Geometry check sheet. Reference: the model listing, model coordinates, mm. Round coordinates to 2 decimals unless told otherwise and drop trailing zeros. Order: outer loops, then holes, each group sorted by start corner. A loop starts at its lowest first (then second) coordinate and runs counter-clockwise, first axis right, second up.
(1) Sectioned sample at A-A (y = 0). Record the boundary of the cut face in (x, z).
(2) Sectioned sample at C-C (z = 2.05). Record the boundary of the cut face in (x, y), plus the area to 3 significant figures.
(3) Release check for a two-part mould opening along Y. For faces 1 (the face through (88.8, 3.4, 4)), 2 (the face through (86, 0, 3)), 3 (the face through (89, 0, 1)), 4 (the face through (180, 0, 2)) record: +Y half, -Y half, draft (parallel to the pull), parting line (faces both ways), or undercut.
(4) Go/stop test with flat-tipped pins: pin 1 (3 mm diameter, centred on x = 105.5, y = 0, fed in from +Z); pin 2 (1.8 mm diameter, centred on x = 48, y = -1, fed in from -Z); pin 3 (1.1 mm diameter, centred on y = 1, z = 3.5, fed in from +X). Record where each tip stops, or that it passes through.
(5) Sectioned sample at B-B (x = 61.5). Record the boundary of the cut face in (y, z), plus the area to 3 significant figures.
(6) Material ranges on line 1 along Y through (x, z) = (0, 1.75); line 2 along Y through (x, z) = (38, 0.25); line 3 along X through (y, z) = (-2, 1.15), recorded low to high.
from build123d import *

# Parameters (mm, degrees)
CROQUIS1_R              = 3.1
SALIENTE_EXTRUIR1_DEPTH = 4
CROQUIS2_W              = 165
CROQUIS2_H              = 6
CORTAR_EXTRUIR1_DEPTH   = 1
CROQUIS3_W              = 165
CROQUIS3_H              = 6
CORTAR_EXTRUIR2_DEPTH   = 1


with BuildPart() as part:
    # Croquis1 → Saliente-Extruir1 (new body)
    with BuildSketch(Plane.XY):
        with BuildLine():
            Line((0, 5), (175, 5))
            ThreePointArc((175, 5), (180, 0), (175, -5))
            Line((175, -5), (0, -5))
            ThreePointArc((0, -5), (-5, 0), (0, 5))
        make_face()
        Circle(CROQUIS1_R, mode=Mode.SUBTRACT)
        with Locations((175, 0)):
            Circle(CROQUIS1_R, mode=Mode.SUBTRACT)
    extrude(amount=SALIENTE_EXTRUIR1_DEPTH)

    # Croquis2 → Cortar-Extruir1 (cut)
    with BuildSketch(Plane.XY.offset(4)):
        with Locations((87.5, 0)):
            Rectangle(CROQUIS2_W, CROQUIS2_H)
    extrude(amount=-CORTAR_EXTRUIR1_DEPTH, mode=Mode.SUBTRACT)

    # Croquis3 → Cortar-Extruir2 (cut)
    with BuildSketch(Plane(origin=(0, 0, 0), x_dir=(-1, 0, 0), z_dir=(0, 0, -1))):
        with Locations((-87.5, 0)):
            Rectangle(CROQUIS3_W, CROQUIS3_H)
    extrude(amount=-CORTAR_EXTRUIR2_DEPTH, mode=Mode.SUBTRACT)


solid = part.part
Answer below:
1. outline: (-5, 0) - (-3.1, 0) - (-3.1, 4) - (-5, 4) - close; (3.1, 0) - (5, 0) - (5, 1) - (170, 1) - (170, 0) - (171.9, 0) - (171.9, 4) - (170, 4) - (170, 3) - (5, 3) - (5, 4) - (3.1, 4) - close; (178.1, 0) - (180, 0) - (180, 4) - (178.1, 4) - close
2. outline: (0, -5) - (175, -5) arc R5 ccw to (175, 5) - (0, 5) arc R5 ccw to start; hole circle Ø6.2 at (0, 0); hole circle Ø6.2 at (175, 0)
2. area: 1,770 mm2
3. face 1: draft
3. face 2: undercut
3. face 3: undercut
3. face 4: parting line
4. pin 1: stops at z = 3
4. pin 2: stops at z = 1
4. pin 3: stops at x = 179.98
5. outline: (-5, 0) - (-3, 0) - (-3, 1) - (3, 1) - (3, 0) - (5, 0) - (5, 4) - (3, 4) - (3, 3) - (-3, 3) - (-3, 4) - (-5, 4) - close
5. area: 28.0 mm2
6. line 1: y = -5 to -3.1, 3.1 to 5
6. line 2: y = -5 to -3, 3 to 5
6. line 3: x = -4.58 to -2.37, 2.37 to 172.63, 177.37 to 179.58
